Source: CAD feature listing. Evaluate the final solid. Frame: model axes, mm. A direction names the side the tool comes from. Give positions to 0.01 mm unless a question says otherwise; leave off trailing zeros. Order: outer loops, then holes, each group sorted by start corner. A loop starts at its lowest first (then second) coordinate and runs counter-clockwise, first axis right, second up. Notation, with made-up numbers: M -18,10.25 L 8,10.25 A9 ccw 8,21.25 Z; hole C 33.25,12 d9. An arc over 180 degrees is marked long. Return JSON: item names as keys, results as strings.
from build123d import *

# Parameters (mm, degrees)
SKETCH1_W           = 120
SKETCH1_H           = 120
BOSS_EXTRUDE1_DEPTH = 10
SKETCH2_R           = 2.75
CUT_EXTRUDE1_DEPTH  = 86.440037453
CIRPATTERN1_COUNT   = 4
FILLET1_R           = 8
FILLET2_R           = 1
SKETCH3_R           = 40
BOSS_EXTRUDE2_DEPTH = 30
SKETCH4_R           = 25.1
CUT_EXTRUDE2_DEPTH  = 25
BOSS_EXTRUDE3_REACH = 95.808
CHAMFER1_SIZE       = 1
FILLET3_R           = 2
FILLET4_R           = 5


with BuildPart() as part:
    # Sketch1 → Boss-Extrude1 (new body)
    with BuildSketch(Plane(origin=(0, 0, 0), x_dir=(1, 0, 0), z_dir=(0, 1, 0))):
        Rectangle(SKETCH1_W, SKETCH1_H)
    extrude(amount=BOSS_EXTRUDE1_DEPTH)

    # Sketch2 → Cut-Extrude1 (cut, through all)
    with BuildSketch(Plane(origin=(0, 10, 0), x_dir=(1, 0, 0), z_dir=(0, 1, 0))):
        with Locations(Location((-52, 52, 0), (0, 0, 270))):
            Circle(SKETCH2_R)
    cut_extrude1 = extrude(amount=-CUT_EXTRUDE1_DEPTH, mode=Mode.SUBTRACT)

    # CirPattern1: Cut-Extrude1 ×4 about axis
    cirpattern1_axis = Axis((0, 0, 0), (0, 1, 0))
    for i in range(1, CIRPATTERN1_COUNT):
        add(cut_extrude1.rotate(cirpattern1_axis, i * 360 / CIRPATTERN1_COUNT), mode=Mode.SUBTRACT)

    # Fillet1
    fillet1_edges = [part.edges().sort_by_distance(p)[0] for p in [
        (60, 5, 60),
        (-60, 5, 60),
        (-60, 5, -60),
        (60, 5, -60),
    ]]
    fillet(fillet1_edges, radius=FILLET1_R)

    # Fillet2
    fillet2_edges = [part.edges().sort_by_distance(p)[0] for p in [
        (0, 10, 60),
        (-60, 10, 0),
        (60, 10, 0),
        (0, 10, -60),
        (-57.656854249, 10, -57.656854249),
        (57.656854249, 10, -57.656854249),
        (57.656854249, 10, 57.656854249),
        (-57.656854249, 10, 57.656854249),
    ]]
    fillet(fillet2_edges, radius=FILLET2_R)

    # Sketch3 → Boss-Extrude2 (add)
    with BuildSketch(Plane(origin=(0, 10, 0), x_dir=(1, 0, 0), z_dir=(0, 1, 0))):
        with Locations(Location((0, 0, 0), (0, 0, 90))):
            Circle(SKETCH3_R)
    extrude(amount=BOSS_EXTRUDE2_DEPTH)

    # Sketch4 → Cut-Extrude2 (cut)
    with BuildSketch(Plane(origin=(0, 40, 0), x_dir=(1, 0, 0), z_dir=(0, 1, 0))):
        with Locations(Location((0, 0, 0), (0, 0, 270))):
            Circle(SKETCH4_R)
    extrude(amount=-CUT_EXTRUDE2_DEPTH, mode=Mode.SUBTRACT)

    # Sketch5 → Boss-Extrude3 (add, up to next)
    with BuildSketch(Plane(origin=(0, 40, 0), x_dir=(1, 0, 0), z_dir=(0, 1, 0)), mode=Mode.PRIVATE) as boss_extrude3_sk1:
        with BuildLine():
            Line((2.9, 21.131907268), (-2.9, 21.131907268))
            Line((-2.9, 21.131907268), (-2.9, 24.931907268))
            ThreePointArc((-2.9, 24.931907268), (0, 25.1), (2.9, 24.931907268))
            Line((2.9, 24.931907268), (2.9, 21.131907268))
        make_face()
    boss_extrude3_tool1 = extrude(boss_extrude3_sk1.sketch, amount=-BOSS_EXTRUDE3_REACH, mode=Mode.PRIVATE) - part.part
    add(boss_extrude3_tool1.solids().sort_by_distance((0, 40, -23.088296))[0])

    # Chamfer1
    chamfer1_edges = [part.edges().sort_by_distance(p)[0] for p in [
        (25.05794158, 40, 1.452433748),
        (-2.9, 40, -23.031907268),
        (0, 40, -21.131907268),
        (2.9, 40, -23.031907268),
    ]]
    chamfer(chamfer1_edges, length=CHAMFER1_SIZE)

    # Fillet3
    fillet3_edges = [part.edges().sort_by_distance(p)[0] for p in [
        (0, 40, 40),
    ]]
    fillet(fillet3_edges, radius=FILLET3_R)

    # Fillet4
    fillet4_edges = [part.edges().sort_by_distance(p)[0] for p in [
        (0, 10, 40),
    ]]
    fillet(fillet4_edges, radius=FILLET4_R)


solid = part.part
1. Section query B-B (z = 0). Return loops of the section in (x, y), then the cut area to 3 significant figures.
Evaluation:
{"outline": "M -60,0 L 60,0 L 60,9 A1 ccw 59,10 L 45,10 A5 cw 40,15 L 40,38 A2 ccw 38,40 L 26.1,40 L 25.1,39 L 25.1,15 L -25.1,15 L -25.1,39 L -26.1,40 L -38,40 A2 ccw -40,38 L -40,15 A5 cw -45,10 L -59,10 A1 ccw -60,9 Z", "area": "2,350 mm^2"}
2. Draft query along X for faces 1 (the face through (0, 15, 0)), 2 (the face through (39.05, 26.34, 8.67)), 3 (the face through (54.027, 5.07, -50.141)), 4 (the face through (-57.719, 4.563, -57.594)). Return one class per face: pulls with the +X half, pulls with the -X half, needs draft (parallel to the pull), parting line crosses it, or undercut.
Evaluation:
{"face 1": "undercut", "face 2": "parting line crosses it", "face 3": "undercut", "face 4": "pulls with the -X half"}
3. Section query A-A (y = 34.5). Return loops of the section in (x, z).
Evaluation:
{"outline": "C 0,0 d80; hole M -2.9,-24.93 L -2.9,-21.13 L 2.9,-21.13 L 2.9,-24.93 A25.1 ccw long Z"}
4. Ray query, probe 1 along X at (y, z) = (2.25, 52); probe 2 along Y at (x, z) = (-2, 53.5); probe 3 along Y at (x, z) = (-3.5, 19). Return the intervals inside material, ascending.
Evaluation:
{"probe 1": "x = -60 to -54.75, -49.25 to 49.25, 54.75 to 60", "probe 2": "y = 0 to 10", "probe 3": "y = 0 to 15"}
5. Set-up query: faces 5 (the face through (-50.141, 5.07, -54.027)), 6 (the face through (-2.9, 27, -23)). Return all of +Z, -Z, +X, -X, +Y, -Y with unobstructed straight access to the full face (end or side cutting, diameter ignored); none if empty.
Evaluation:
{"face 5": "+Y, -Y", "face 6": "+Y"}
6. First-contact query: pin 1 (3 mm diameter, centred on y = 26, z = -23.5, fed in from +X); pin 2 (25 mm diameter, centred on x = -8.5, z = 5.5, fed in from +Y); pin 3 (1 mm diameter, centred on y = 24, z = -2, fed in from +X). Flat tips, straight axial feed; report the tip coordinate or a pass-through.
Evaluation:
{"pin 1": "stops at x = 33.41", "pin 2": "stops at y = 15", "pin 3": "stops at x = 39.97"}
